The listing builds one solid part. Answer for the finished solid, in the listing's coordinates (mm). A direction names the side the tool comes from. Give positions to 0.01 mm unless a question says otherwise; leave off trailing zeros. Write each loop counter-clockwise with the first axis right and the second up, starting at its lowest first coordinate (ties: lowest second). Pieces come first, ordered by that corner, then holes.
```python
from build123d import *

# Parameters (mm, degrees)
F0_W      = 86
F0_H      = 30
F0_R      = 8.35
F1_DEPTH  = 12.5
F3_DEPTH  = 12.5
F4_R      = 1.65
F5_DEPTH  = 65
F6_R      = 1.65
F7_DEPTH  = 12.5
F9_DEPTH  = 12.5
F11_DEPTH = 12.5
F13_DEPTH = 3
F14_R     = 2.15
F15_DEPTH = 12.5


with BuildPart() as f1:
    # F0 (on Front) → F1 (new body, symmetric)
    with BuildSketch(Plane.XZ):
        Rectangle(F0_W, F0_H)
        Circle(F0_R, mode=Mode.SUBTRACT)
    extrude(amount=F1_DEPTH, both=True)

    # F2 (on Front) → F3 (cut, symmetric)
    with BuildSketch(Plane.XZ):
        with BuildLine():
            Line((38, 15), (-38, 15))
            Line((-38, 15), (-38, 5))
            Line((-38, 5), (-13, 5))
            ThreePointArc((-13, 5), (0, 13.9283882772), (13, 5))
            Line((13, 5), (38, 5))
            Line((38, 5), (38, 15))
        make_face()
        with BuildLine():
            Line((-13, -5), (-38, -5))
            Line((-38, -5), (-38, -15))
            Line((-38, -15), (38, -15))
            Line((38, -15), (38, -5))
            Line((38, -5), (13, -5))
            ThreePointArc((13, -5), (0, -13.9283882772), (-13, -5))
        make_face()
    extrude(amount=F3_DEPTH, both=True, mode=Mode.SUBTRACT)

    # F4 (on Right) → F5 (cut, symmetric)
    with BuildSketch(Plane.YZ):
        with Locations((8.5, 11)):
            Circle(F4_R)
        with Locations((8.5, -11)):
            Circle(F4_R)
        with Locations((-8.5, 11)):
            Circle(F4_R)
        with Locations((-8.5, -11)):
            Circle(F4_R)
    extrude(amount=F5_DEPTH, both=True, mode=Mode.SUBTRACT)

    # F6 (on Right) → F7 (join, symmetric)
    with BuildSketch(Plane.YZ):
        with Locations((8.5, 11)):
            Circle(F6_R)
        with Locations((8.5, -11)):
            Circle(F6_R)
        with Locations((-8.5, 11)):
            Circle(F6_R)
        with Locations((-8.5, -11)):
            Circle(F6_R)
    extrude(amount=F7_DEPTH, both=True)

    # F8 (on Front) → F9 (cut, symmetric)
    with BuildSketch(Plane.XZ):
        with BuildLine():
            Line((38, 15), (-38, 15))
            Line((-38, 15), (-38, 5))
            Line((-38, 5), (-13, 5))
            ThreePointArc((-13, 5), (0, 13.9283882772), (13, 5))
            Line((13, 5), (38, 5))
            Line((38, 5), (38, 15))
        make_face()
        with BuildLine():
            Line((-13, -5), (-38, -5))
            Line((-38, -5), (-38, -15))
            Line((-38, -15), (38, -15))
            Line((38, -15), (38, -5))
            Line((38, -5), (13, -5))
            ThreePointArc((13, -5), (0, -13.9283882772), (-13, -5))
        make_face()
    extrude(amount=F9_DEPTH, both=True, mode=Mode.SUBTRACT)

    # F10 (on Front) → F11 (cut, symmetric)
    with BuildSketch(Plane.XZ):
        with BuildLine():
            ThreePointArc((0.75, 13.9081810457), (0, 14.6581810457), (-0.75, 13.9081810457))
            Line((-0.75, 13.9081810457), (-0.75, 8.3162491545))
            ThreePointArc((-0.75, 8.3162491545), (0, 7.5662491545), (0.75, 8.3162491545))
            Line((0.75, 8.3162491545), (0.75, 13.9081810457))
        make_face()
    extrude(amount=F11_DEPTH, both=True, mode=Mode.SUBTRACT)

    # F12 (on Front) → F13 (join, symmetric)
    with BuildSketch(Plane.XZ):
        with BuildLine():
            Line((-0.75, 13.9081810457), (-0.75, 18.6542118044))
            Line((-0.75, 18.6542118044), (-2.75, 18.6542118044))
            Line((-2.75, 18.6542118044), (-2.75, 13.6542118044))
            ThreePointArc((-2.75, 13.6542118044), (-1.754601121, 13.8174301122), (-0.75, 13.9081810457))
        make_face()
        with BuildLine():
            Line((0.75, 18.6542118044), (0.75, 13.9081810457))
            ThreePointArc((0.75, 13.9081810457), (1.754601121, 13.8174301122), (2.75, 13.6542118044))
            Line((2.75, 13.6542118044), (2.75, 18.6542118044))
            Line((2.75, 18.6542118044), (0.75, 18.6542118044))
        make_face()
    extrude(amount=F13_DEPTH, both=True)

    # F14 (on Right) → F15 (cut, symmetric)
    with BuildSketch(Plane.YZ):
        with Locations((0, 16.1542118044)):
            Circle(F14_R)
    extrude(amount=F15_DEPTH, both=True, mode=Mode.SUBTRACT)


solid = f1.part
```
Item 1: A cutting plane is placed at B-B, the plane y = 0. Count the separate pieces of the cut face and the enclosed holes in it, plus the area to 3 significant figures.
Conclusion:
separate pieces: 3
enclosed holes: 0
area: 1,170 mm2
Item 2: A cutting plane is placed at C-C, the plane x = 4.5. Give the vertices of the cut face in (y, z).
Conclusion:
outline: (-12.5, -13.18) - (12.5, -13.18) - (12.5, -7.03) - (-12.5, -7.03) - close; (-12.5, 7.03) - (12.5, 7.03) - (12.5, 13.18) - (-12.5, 13.18) - close
Item 3: Each of these flat-tipped pins is pushed along its axis until it touches: P1, Ø10, axis at x = -7, y = -9.5, coming from the -Z side; P2, Ø2, axis at x = -1.5, z = 15.5, coming from the -Y side; P3, Ø1.6, axis at x = 1.5, z = 15, coming from the +Y side. Where does it stop, or does it pass through?
Conclusion:
P1: stops at z = -13.78
P2: stops at y = -3
P3: stops at y = 3
Item 4: Consider probe 1 along Y at (x, z) = (41, 11); probe 2 along Z at (x, y) = (39.4, -8.5); probe 3 along X at (y, z) = (9.5, 7). Determine where each line is inside the solid, lowest interval first.
Conclusion:
probe 1: y = -12.5 to -10.15, -6.85 to 6.85, 10.15 to 12.5
probe 2: z = -15 to -12.65, -9.35 to 9.35, 12.65 to 15
probe 3: x = -43 to -38, -12.04 to -4.55, 4.55 to 12.04, 38 to 43
Item 5: Which of the six approach directions +Z, -Z, +X, -X, +Y, -Y give full straight-line access (tool end or side, diameter ignored) to faces 1 (the face through (-38, 0, 10)), 2 (the face through (-40.47, 7.19, -12)), 3 (the face through (1.764, 1.156, 17.967)), 4 (the face through (40.47, -9.81, 10))?
Conclusion:
face 1: +Z, +Y, -Y
face 2: -X
face 3: none
face 4: +X
Item 6: A cutting plane is placed at D-D, the plane y = 4.25. Give the vertices of the cut face in (x, z).
Conclusion:
outline: (-43, -15) - (-38, -15) - (-38, -5) - (-13, -5) arc R13.93 ccw to (13, -5) - (38, -5) - (38, -15) - (43, -15) - (43, 15) - (38, 15) - (38, 5) - (13, 5) arc R13.93 ccw to (0.75, 13.91) - (0.75, 8.32) arc R8.35 cw (long way) to (-0.75, 8.32) - (-0.75, 13.91) arc R13.93 ccw to (-13, 5) - (-38, 5) - (-38, 15) - (-43, 15) - close
Item 7: Determine the mould class of faces 5 (the face through (-40.47, -9.81, 10)), 6 (the face through (25, 0, 5)), 7 (the face through (-10, 12.5, 0)) for opening direction Y: pulls with the +Y half, pulls with the -Y half, needs draft (parallel to the pull), parting line crosses it, or undercut.
Conclusion:
face 5: undercut
face 6: needs draft
face 7: pulls with the +Y half
Item 8: A cutting plane is placed at A-A, the plane z = 0. Give the vertices of the cut face in (x, y).
Conclusion:
outline: (-43, -12.5) - (-8.35, -12.5) - (-8.35, 12.5) - (-43, 12.5) - close; (8.35, -12.5) - (43, -12.5) - (43, 12.5) - (8.35, 12.5) - close
